```python
from build123d import *

# Parameters (mm, degrees)
ESQUISSE1_W             = 20
ESQUISSE1_H             = 30
BOSS_EXTRU_1_DEPTH      = 10
ESQUISSE2_R             = 6
BOSS_EXTRU_2_DEPTH      = 40
ESQUISSE3_W             = 40
ESQUISSE3_H             = 30
BOSS_EXTRU_3_DEPTH      = 15
ESQUISSE4_R             = 4.5
ENL_V_MAT_EXTRU_1_DEPTH = 55
ENL_V_MAT_EXTRU_3_DEPTH = 55


with BuildPart() as part:
    # Esquisse1 → Boss.-Extru.1 (new body)
    with BuildSketch(Plane.XY):
        with Locations((-10, 15)):
            Rectangle(ESQUISSE1_W, ESQUISSE1_H)
    extrude(amount=BOSS_EXTRU_1_DEPTH)

    # Esquisse2 → Boss.-Extru.2 (add)
    with BuildSketch(Plane.XY.offset(10)):
        with Locations((-10, 18)):
            Circle(ESQUISSE2_R)
    extrude(amount=BOSS_EXTRU_2_DEPTH)

    # Esquisse3 → Boss.-Extru.3 (add)
    with BuildSketch(Plane.XZ):
        with Locations((-10, 15)):
            Rectangle(ESQUISSE3_W, ESQUISSE3_H)
    extrude(amount=BOSS_EXTRU_3_DEPTH)

    # Esquisse4 → Enlèv. mat.-Extru.1 (cut)
    with BuildSketch(Plane(origin=(0, 0, 0), x_dir=(-1, 0, 0), z_dir=(0, 0, -1))):
        with Locations((10, -15)):
            Circle(ESQUISSE4_R)
    extrude(amount=-ENL_V_MAT_EXTRU_1_DEPTH, mode=Mode.SUBTRACT)

    # Esquisse5 → Enlèv. mat.-Extru.3 (cut)
    with BuildSketch(Plane(origin=(0, 0, 0), x_dir=(-1, 0, 0), z_dir=(0, 0, -1))):
        with BuildLine():
            Line((30, 0), (25, 0))
            ThreePointArc((25, 0), (28.535533906, -1.464466094), (30, -5))
            Line((30, -5), (30, 0))
        make_face()
        with BuildLine():
            Line((-10, 0), (-10, -5))
            ThreePointArc((-10, -5), (-8.535533906, -1.464466094), (-5, 0))
            Line((-5, 0), (-10, 0))
        make_face()
    extrude(amount=-ENL_V_MAT_EXTRU_3_DEPTH, mode=Mode.SUBTRACT)


solid = part.part
```
Geometry: final body of the model. Coordinates: model frame, mm. A direction names the side the tool comes from. Coordinates: 2 decimals unless noted, no trailing zeros. Loops run counter-clockwise (first coordinate to the right, second up) from the corner with the lowest first, then second, coordinate; pieces in that order, holes last. Notation, with made-up numbers: M -33,30 L 12,30 A18 ccw 12,60 Z; hole C 62.5,18.25 d11. An arc over 180 degrees is marked long. Put each result on its own line as item: value.
(1) Cut plane B-B on z = 17.5. Return the cut outline in (x, y).
Answer sheet:
outline: M -30,-15 L -14.5,-15 A4.5 cw -5.5,-15 L 10,-15 L 10,-5 A5 ccw 5,0 L -25,0 A5 ccw -30,-5 Z; C -10,18 d12
(2) Cut plane D-D on z = 42.5. Return the cut outline in (x, y).
Answer sheet:
outline: C -10,18 d12
(3) Cut plane A-A on x = -10. Return the cut outline in (y, z).
Answer sheet:
outline: M -10.5,0 L 30,0 L 30,10 L 24,10 L 24,50 L 12,50 L 12,10 L 0,10 L 0,30 L -10.5,30 Z
(4) Draft query along Y for faces 4 (the face through (10, -10, 15)), 5 (the face through (-10, 30, 5)), 6 (the face through (-4.277, 19.802, 29.72)), 7 (the face through (2, -15, 15)). Return one class per face: pulls with the +Y half, pulls with the -Y half, needs draft (parallel to the pull), parting line crosses it, or undercut.
Answer sheet:
face 4: needs draft
face 5: pulls with the +Y half
face 6: undercut
face 7: pulls with the -Y half
(5) Access query for faces 1 (the face through (0, 15, 5)), 2 (the face through (-20, 15, 5)), 3 (the face through (-10, -7, 30)). Directions: +Z, -Z, +X, -X, +Y, -Y. A direction counts if a zero-diameter tool reaches every point of the face in a straight line with its end or side. Return the directions, or none.
Answer sheet:
face 1: +Z, -Z, +X, +Y
face 2: +Z, -Z, -X, +Y
face 3: +Z, +X, -X, -Y
(6) First-contact query: pin 1 (4 mm diameter, centred on x = -9, z = 38.5, fed in from +Y); pin 2 (10 mm diameter, centred on x = -3, z = 30.5, fed in from +Y); pin 3 (1 mm diameter, centred on x = -19.5, y = -9, fed in from +Z). Flat tips, straight axial feed; report the tip coordinate or a pass-through.
Answer sheet:
pin 1: stops at y = 24
pin 2: stops at y = 23.66
pin 3: stops at z = 30
(7) Cut plane C-C on y = 18. Return the cut outline in (x, z), then the cut area to 3 significant figures.
Answer sheet:
outline: M -20,0 L 0,0 L 0,10 L -4,10 L -4,50 L -16,50 L -16,10 L -20,10 Z
area: 680 mm^2
(8) Material intervals for probe 1 along Z at (x, y) = (-6, -7); probe 2 along Z at (x, y) = (-11.5, 2); probe 3 along Y at (x, z) = (3, 25), sorted ascending.
Answer sheet:
probe 1: z = 0 to 30
probe 2: z = 0 to 10
probe 3: y = -15 to 0
